Here's how the part is built. I have some questions about the finished solid (model axes, mm). Give positions to 0.01 mm unless a question says otherwise; leave off trailing zeros. Loops run counter-clockwise (first coordinate to the right, second up) from the corner with the lowest first, then second, coordinate; pieces in that order, holes last.
Q1. Thinking about a two-plate mould opening in Z: for faces 1 (the face through (0.91, 12.87, 30.61)), 2 (the face through (57.1, 4, -26.1)), 3 (the face through (1, 21.6, 0)), which applies, pulls with the +Z half, pulls with the -Z half, needs draft (parallel to the pull), parting line crosses it, or undercut?
Q2. Suppose I cut it at A-A (x = -42.5). List the corners of the cut face in (y, z) for me.
Q3. I need wall thicknesses on probe 1 along X at (y, z) = (1, 37.5); probe 2 along Z at (x, y) = (-40, 0.9); probe 3 along Z at (x, y) = (-27.5, 1.25). Which ranges of each line are inside material? Lowest first, please.
Q4. Suppose I cut it at B-B (y = 6.5). Count the separate pieces of the cut face and the enclosed holes in it, and give its area (3 significant figures).
Q5. I'm going to push flat-ended pins straight in: P1, Ø12, axis at x = 41.5, y = 17, coming from the +Z side; P2, Ø5, axis at x = -47.5, z = 6, coming from the -Y side; P3, Ø4.5, axis at x = 56, z = -23.5, coming from the -Y side; P4, Ø1.2, axis at x = 39.5, z = 38, coming from the -Y side. Where does each tip first touch, or does it pass through?
```python
from build123d import *

# Parameters (mm, degrees)
SKETCH1_W               = 130
SKETCH1_H               = 82
BOSS_EXTRUDE1_DEPTH     = 5
SKETCH3_W               = 130
SKETCH3_H               = 82
SKETCH2_W               = 120
SKETCH2_H               = 46
CHAMFER1_SIZE           = 2
SKETCH4_R               = 1.2
CUT_EXTRUDE1_DEPTH      = 4
SKETCH5_W               = 114
SKETCH5_H               = 40
CUT_EXTRUDE2_DEPTH      = 21
SKETCH6_W               = 118
SKETCH6_H               = 56
CUT_EXTRUDE3_DEPTH      = 12
SKETCH8_W               = 7
SKETCH8_H               = 7
BOSS_EXTRUDE2_DEPTH     = 8
SKETCH9_R               = 2.1
CUT_EXTRUDE4_DEPTH      = 8
SKETCH10_W              = 2
SKETCH10_H              = 40
CUT_EXTRUDE5_DEPTH      = 9
CUT_EXTRUDE6_DEPTH      = 66.0000001
CUT_EXTRUDE6_DEPTH_BACK = 66.0000001
SKETCH12_W              = 82
SKETCH12_H              = 2
CUT_EXTRUDE7_DEPTH      = 66.0000001
CUT_EXTRUDE7_DEPTH_BACK = 66.0000001
FILLET1_R               = 3
CHAMFER2_SIZE           = 0.4


with BuildPart() as part:
    # Sketch1 → Boss-Extrude1 (new body)
    with BuildSketch(Plane(origin=(0, 0, 0), x_dir=(1, 0, 0), z_dir=(0, 1, 0))):
        Rectangle(SKETCH1_W, SKETCH1_H)
    extrude(amount=BOSS_EXTRUDE1_DEPTH)

    # Sketch3 → Loft2 section 0
    with BuildSketch(Plane(origin=(0, 5, 0), x_dir=(1, 0, 0), z_dir=(0, 1, 0))):
        Rectangle(SKETCH3_W, SKETCH3_H)
    # Sketch2 → Loft2 section 1
    with BuildSketch(Plane(origin=(0, 22, 0), x_dir=(1, 0, 0), z_dir=(0, 1, 0))):
        Rectangle(SKETCH2_W, SKETCH2_H)
    loft()

    # Chamfer1
    chamfer1_edges = [part.edges().sort_by_distance(p)[0] for p in [
        (-65, 2.5, 41),
        (65, 2.5, 41),
        (65, 2.5, -41),
        (-65, 2.5, -41),
    ]]
    chamfer(chamfer1_edges, length=CHAMFER1_SIZE)

    # Sketch4 → Cut-Extrude1 (cut)
    with BuildSketch(Plane.XZ):
        with Locations((40, -37.5)):
            Circle(SKETCH4_R)
        with Locations((-40, -37.5)):
            Circle(SKETCH4_R)
    cut_extrude1 = extrude(amount=-CUT_EXTRUDE1_DEPTH, mode=Mode.SUBTRACT)

    # Sketch5 → Cut-Extrude2 (cut)
    with BuildSketch(Plane.XZ):
        Rectangle(SKETCH5_W, SKETCH5_H)
    extrude(amount=-CUT_EXTRUDE2_DEPTH, mode=Mode.SUBTRACT)

    # Mirror1: Cut-Extrude1 across plane
    add(cut_extrude1.mirror(Plane.XY), mode=Mode.SUBTRACT)

    # Sketch6 → Cut-Extrude3 (cut)
    with BuildSketch(Plane.XZ):
        Rectangle(SKETCH6_W, SKETCH6_H)
    extrude(amount=-CUT_EXTRUDE3_DEPTH, mode=Mode.SUBTRACT)

    # Sketch8 → Boss-Extrude2 (add)
    with BuildSketch(Plane(origin=(0, 4, 0), x_dir=(-1, 0, 0), z_dir=(0, -1, 0))):
        with Locations((-55.5, 24.5)):
            Rectangle(SKETCH8_W, SKETCH8_H)
        with Locations((-55.5, -24.5)):
            Rectangle(SKETCH8_W, SKETCH8_H)
        with Locations((55.5, -24.5)):
            Rectangle(SKETCH8_W, SKETCH8_H)
        with Locations((55.5, 24.5)):
            Rectangle(SKETCH8_W, SKETCH8_H)
    extrude(amount=-BOSS_EXTRUDE2_DEPTH)

    # Sketch9 → Cut-Extrude4 (cut)
    with BuildSketch(Plane.XZ.offset(-4)):
        with Locations((-55.5, 24.5)):
            Circle(SKETCH9_R)
        with Locations((55.5, 24.5)):
            Circle(SKETCH9_R)
        with Locations((55.5, -24.5)):
            Circle(SKETCH9_R)
        with Locations((-55.5, -24.5)):
            Circle(SKETCH9_R)
    extrude(amount=-CUT_EXTRUDE4_DEPTH, mode=Mode.SUBTRACT)

    # Sketch10 → Cut-Extrude5 (cut)
    with BuildSketch(Plane.XZ.offset(-12)):
        with Locations((-58, 0)):
            Rectangle(SKETCH10_W, SKETCH10_H)
        with Locations((58, 0)):
            Rectangle(SKETCH10_W, SKETCH10_H)
    extrude(amount=-CUT_EXTRUDE5_DEPTH, mode=Mode.SUBTRACT)

    # Sketch11 → Cut-Extrude6 (cut, two sides)
    with BuildSketch(Plane(origin=(0, 0, 0), x_dir=(0, 0, -1), z_dir=(1, 0, 0))) as cut_extrude6_sk:
        Polygon((21, 22), (41, 3), (41, 5), (23, 22), align=None)
        Polygon((-23, 22), (-21, 22), (-41, 3), (-41, 5), align=None)
    extrude(amount=CUT_EXTRUDE6_DEPTH, mode=Mode.SUBTRACT)
    extrude(cut_extrude6_sk.sketch, amount=-CUT_EXTRUDE6_DEPTH_BACK, mode=Mode.SUBTRACT)

    # Sketch12 → Cut-Extrude7 (cut, two sides)
    with BuildSketch(Plane(origin=(0, 0, 0), x_dir=(0, 0, -1), z_dir=(1, 0, 0))) as cut_extrude7_sk:
        with Locations((0, 22.6)):
            Rectangle(SKETCH12_W, SKETCH12_H)
    extrude(amount=CUT_EXTRUDE7_DEPTH, mode=Mode.SUBTRACT)
    extrude(cut_extrude7_sk.sketch, amount=-CUT_EXTRUDE7_DEPTH_BACK, mode=Mode.SUBTRACT)

    # Fillet1
    fillet1_edges = [part.edges().sort_by_distance(p)[0] for p in [
        (0, 3, -41),
        (0, 3, 41),
    ]]
    fillet(fillet1_edges, radius=FILLET1_R)

    # Chamfer2
    chamfer2_edges = [part.edges().sort_by_distance(p)[0] for p in [
        (0, 0, 41),
        (65, 0, 0),
        (-65, 0, 0),
        (0, 0, -41),
        (-64, 0, -40),
        (64, 0, -40),
        (64, 0, 40),
        (-64, 0, 40),
    ]]
    chamfer(chamfer2_edges, length=CHAMFER2_SIZE)


solid = part.part
```
Solutions:
1. face 1: pulls with the +Z half
1. face 2: undercut
1. face 3: needs draft
2. outline: (0, -40.6) - (0.4, -41) - (1.71, -41) arc R3 ccw to (3.89, -40.07) - (21.6, -21.42) - (21.6, 21.42) - (3.89, 40.07) arc R3 ccw to (1.71, 41) - (0.4, 41) - (0, 40.6) - (0, 28) - (12, 28) - (12, 20) - (21, 20) - (21, -20) - (12, -20) - (12, -28) - (0, -28) - close
3. probe 1: x = -65 to -41.2, -38.8 to 38.8, 41.2 to 65
3. probe 2: z = -41 to -38.7, -36.3 to -28, 28 to 36.3, 38.7 to 41
3. probe 3: z = -41 to -28, 28 to 41
4. separate pieces: 1
4. enclosed holes: 5
4. area: 3,170 mm2
5. P1: stops at z = 32.58
5. P2: stops at y = 21
5. P3: stops at y = 4
5. P4: stops at y = 0
